Verification items for this drawing (mm, ordinates from the low corner). A direction names the side the tool comes from. Coordinates: 2 decimals unless noted, no trailing zeros. Order: outer loops, then holes, each group sorted by start corner. A loop starts at its lowest first (then second) coordinate and runs counter-clockwise, first axis right, second up.
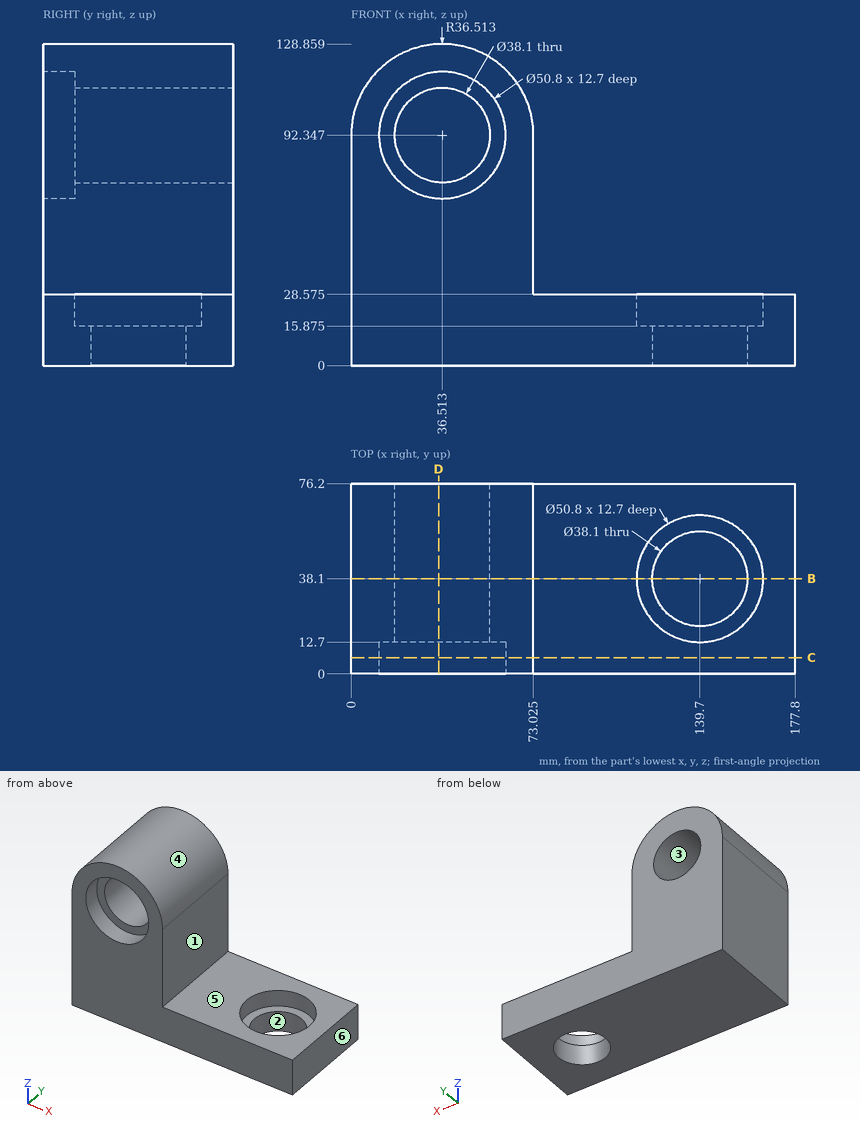
Item 1: Sectioned sample at B-B (y = 38.1). Give the number of separate pieces and of enclosed holes in the cut face, and give its area (3 significant figures).
Item 2: Release check for a two-part mould opening along X. For the marked faces 1, 2, 3 and 4 record: pulls with the +X half, pulls with the -X half, needs draft (parallel to the pull), parting line crosses it, or undercut.
Item 3: Tool access check on the marked faces 5 and 6. Record the directions out of +Z, -Z, +X, -X, +Y, -Y that give a thin tool (end or side, any length) a straight path to the whole face; none if there is none.
Item 4: Depth check by flat-ended pin: P1, Ø3, axis at x = 112.5, y = 49, coming from the +Z side (1 decimal); P2, Ø23, axis at x = 36.51, z = 92.35, coming from the +Y side; P3, Ø1.5, axis at y = 19.5, z = 85.5, coming from the +X side (1 decimal). Enter the tip coordinate at first touch or a pass-through.
Item 5: Sectioned sample at C-C (y = 6.5). Record the cut outline in (x, z) (1 decimal).
Item 6: Sectioned sample at D-D (x = 35). Record the cut outline in (y, z), and give its area (3 significant figures).
Item 7: Thickness scan on line 1 along Z through (x, y) = (37.5, 32) (1 decimal); line 2 along Y through (x, z) = (139.5, 26.5); line 3 along Z through (x, y) = (117, 6) (1 decimal). Record the ranges inside material, lowest first.
Geometry check:
1. separate pieces: 2
1. enclosed holes: 1
1. area: 9,440 mm2
2. face 1: pulls with the +X half
2. face 2: undercut
2. face 3: undercut
2. face 4: parting line crosses it
3. face 5: +Z, +X, +Y, -Y
3. face 6: +Z, -Z, +X, +Y, -Y
4. P1: stops at z = 28.6
4. P2: passes through
4. P3: stops at x = 73
5. outline: (0, 0) - (177.8, 0) - (177.8, 28.6) - (73, 28.6) - (73, 92.3) arc R36.5 ccw to (0, 92.3) - close; hole circle Ø50.8 at (36.5, 92.3)
6. outline: (0, 0) - (76.2, 0) - (76.2, 73.36) - (12.7, 73.36) - (12.7, 66.99) - (0, 66.99) - close; (0, 117.7) - (12.7, 117.7) - (12.7, 111.34) - (76.2, 111.34) - (76.2, 128.83) - (0, 128.83) - close
6. area: 6,760 mm2
7. line 1: z = 0 to 73.3, 111.4 to 128.8
7. line 2: y = 0 to 12.7, 63.5 to 76.2
7. line 3: z = 0 to 28.6
